Part model, mm, in its own coordinate system. Face numbers are marked on the shaded views. A direction names the side the tool comes from. Coordinates: 2 decimals unless noted, no trailing zeros. Write each loop counter-clockwise with the first axis right and the second up, starting at its lowest first coordinate (ties: lowest second). Pieces come first, ordered by that corner, then holes. Notation, with made-up numbers: (1, 8.25) - (18, 8.25) arc R19 ccw to (18, 26.25) - close; hole circle Ø1 at (7, -20.5). An arc over 180 degrees is marked (long way). Use a Markdown table: item, result.
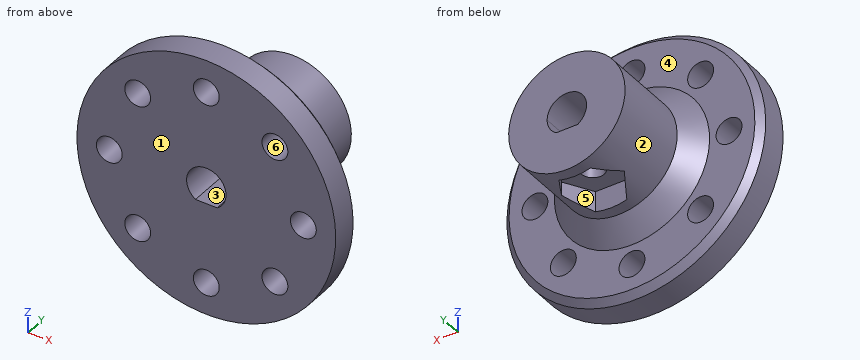
```python
from build123d import *

# Parameters (mm, degrees)
SKETCH1_R           = 20
BOSS_EXTRUDE1_DEPTH = 5
SKETCH2_R           = 2
CUT_EXTRUDE1_DEPTH  = 29.722813233
SKETCH3_R           = 9
BOSS_EXTRUDE2_DEPTH = 15
CUT_EXTRUDE2_DEPTH  = 35.641016151
CHAMFER3_SIZE       = 3
CHAMFER4_SIZE       = 1
SKETCH10_R          = 1.75
CUT_EXTRUDE7_DEPTH  = 3.5
CUT_EXTRUDE8_REACH  = 42.509
SKETCH10_3_R        = 1.75


with BuildPart() as part:
    # Sketch1 → Boss-Extrude1 (new body)
    with BuildSketch(Plane(origin=(0, 0, 0), x_dir=(1, 0, 0), z_dir=(0, 1, 0))):
        with Locations(Location((0, 0, 0), (0, 0, 270))):
            Circle(SKETCH1_R)
    extrude(amount=BOSS_EXTRUDE1_DEPTH)

    # Sketch2 → Cut-Extrude1 (cut, through all)
    with BuildSketch(Plane(origin=(0, 5, 0), x_dir=(1, 0, 0), z_dir=(0, 1, 0))):
        with Locations(Location((0, 15, 0), (0, 0, 270))):
            Circle(SKETCH2_R)
        with Locations(Location((10.606601718, 10.606601718, 0), (0, 0, 270))):
            Circle(SKETCH2_R)
        with Locations(Location((15, 0, 0), (0, 0, 270))):
            Circle(SKETCH2_R)
        with Locations(Location((10.606601718, -10.606601718, 0), (0, 0, 270))):
            Circle(SKETCH2_R)
        with Locations(Location((0, -15, 0), (0, 0, 270))):
            Circle(SKETCH2_R)
        with Locations(Location((-10.606601718, -10.606601718, 0), (0, 0, 270))):
            Circle(SKETCH2_R)
        with Locations(Location((-15, 0, 0), (0, 0, 270))):
            Circle(SKETCH2_R)
        with Locations(Location((-10.606601718, 10.606601718, 0), (0, 0, 270))):
            Circle(SKETCH2_R)
    extrude(amount=-CUT_EXTRUDE1_DEPTH, mode=Mode.SUBTRACT)

    # Sketch3 → Boss-Extrude2 (add)
    with BuildSketch(Plane(origin=(0, 5, 0), x_dir=(1, 0, 0), z_dir=(0, 1, 0))):
        with Locations(Location((0, 0, 0), (0, 0, 270))):
            Circle(SKETCH3_R)
    extrude(amount=BOSS_EXTRUDE2_DEPTH)

    # Sketch4 → Cut-Extrude2 (cut, through all)
    with BuildSketch(Plane(origin=(0, 20, 0), x_dir=(1, 0, 0), z_dir=(0, 1, 0))):
        with BuildLine():
            Line((1.673320053, 2.55), (-1.673320053, 2.55))
            ThreePointArc((-1.673320053, 2.55), (-1.44894338, -2.683852284), (3.05, 0))
            ThreePointArc((3.05, 0), (2.683852284, 1.44894338), (1.673320053, 2.55))
        make_face()
    extrude(amount=-CUT_EXTRUDE2_DEPTH, mode=Mode.SUBTRACT)

    # Chamfer3
    chamfer3_edges = [part.edges().sort_by_distance(p)[0] for p in [
        (0, 5, -9),
    ]]
    chamfer(chamfer3_edges, length=CHAMFER3_SIZE)

    # Chamfer4
    chamfer4_edges = [part.edges().sort_by_distance(p)[0] for p in [
        (0, 5, -20),
    ]]
    chamfer(chamfer4_edges, length=CHAMFER4_SIZE)

    # Sketch10 → Cut-Extrude7 (cut)
    # profile 1 of 2: a face of its own
    with BuildSketch(Plane(origin=(0, 0, -9), x_dir=(-1, 0, 0), z_dir=(0, 0, -1))):
        Polygon((2.424871131, 9.8), (4.849742261, 14), (2.424871131, 18.2), (-2.424871131, 18.2), (-4.849742261, 14), (-2.424871131, 9.8), align=None)
        with Locations((0, 14)):
            Circle(SKETCH10_R, mode=Mode.SUBTRACT)
    # profile 2 of 2: a face of its own
    with BuildSketch(Plane(origin=(0, 0, -9), x_dir=(-1, 0, 0), z_dir=(0, 0, -1))):
        with Locations((0, 14)):
            Circle(SKETCH10_R)
    extrude(amount=-CUT_EXTRUDE7_DEPTH, mode=Mode.SUBTRACT)

    # Sketch10_3 → Cut-Extrude8 (cut, up to next)
    with BuildSketch(Plane(origin=(0, 0, -9), x_dir=(-1, 0, 0), z_dir=(0, 0, -1)), mode=Mode.PRIVATE) as cut_extrude8_sk1:
        with Locations((0, 14)):
            Circle(SKETCH10_3_R)
    cut_extrude8_tool1 = extrude(cut_extrude8_sk1.sketch, amount=-CUT_EXTRUDE8_REACH, mode=Mode.PRIVATE) & part.part
    add(cut_extrude8_tool1.solids().sort_by_distance((0, 14, -9))[0], mode=Mode.SUBTRACT)


solid = part.part
```
Item 1: Two-plate mould, pull along X, no slides. Class the marked faces 1, 2 and 3: pulls with the +X half, pulls with the -X half, needs draft (parallel to the pull), parting line crosses it, or undercut.
From the geometry:
| item | result |
|---|---|
| face 1 | needs draft |
| face 2 | parting line crosses it |
| face 3 | undercut |
Item 2: Drop flat-ended pins along their axis: P1, Ø4, axis at y = 3.5, z = -7, coming from the -X side; P2, Ø6, axis at x = -1, y = 10.5, coming from the +Z side; P3, Ø2, axis at x = 0, y = 14, coming from the -Z side; P4, Ø5, axis at x = 0, z = 0, coming from the -Y side. Give the stop position or say it passes through.
From the geometry:
| item | result |
|---|---|
| P1 | x = -19.36 |
| P2 | z = 9.46 |
| P3 | z = 2.88 |
| P4 | through |
Item 3: Which spindle directions (+Z, -Z, +X, -X, +Y, -Y) get a long thin tool onto all of the face, cutting with end or side? Do the marked faces 4, 5 and 6. Say none if no direction does.
From the geometry:
| item | result |
|---|---|
| face 4 | +Y |
| face 5 | -Z |
| face 6 | +Y, -Y |
Item 4: Band-saw the part on A-A, the plane x = 0. Count the separate pieces of the cut face and the enclosed holes in it, then the cut area to 3 significant figures.
From the geometry:
| item | result |
|---|---|
| separate pieces | 5 |
| enclosed holes | 0 |
| area | 286 mm^2 |
Item 5: Drill centre lines: probe 1 along Y at (x, z) = (0, -4); probe 2 along Y at (x, z) = (-11, -14); probe 3 along Z at (x, y) = (-9.5, 2). Where is each one in solid material? Low to high.
From the geometry:
| item | result |
|---|---|
| probe 1 | 0 to 12.25, 15.75 to 20 |
| probe 2 | 0 to 5 |
| probe 3 | -17.6 to -12.27, -8.94 to 8.94, 12.27 to 17.6 |
Item 6: Band-saw the part on B-B, the plane y = 6.5. Give the cut face in (x, z).
From the geometry:
| item | result |
|---|---|
| outline | circle Ø21 at (0, 0); hole (-1.67, -2.55) - (1.67, -2.55) arc R3.05 ccw (long way) to start |
